from build123d import *

# Parameters (mm, degrees)
SALIENTE_EXTRUIR1_DEPTH = 120
CROQUIS2_R              = 1.5
CORTAR_EXTRUIR1_DEPTH   = 100
CROQUIS3_R              = 1.5
CORTAR_EXTRUIR2_DEPTH   = 100


with BuildPart() as part:
    # Croquis1 → Saliente-Extruir1 (new body)
    with BuildSketch(Plane.XY):
        Polygon((0, 0), (50.8, 0), (50.8, 3.175), (3.175, 3.175), (3.175, 50.8), (0, 50.8), align=None)
    extrude(amount=SALIENTE_EXTRUIR1_DEPTH)

    # Croquis2 → Cortar-Extruir1 (cut)
    with BuildSketch(Plane(origin=(0, 3.175, 0), x_dir=(1, 0, 0), z_dir=(0, 1, 0))):
        with Locations(Location((40.8, -29.9, 0), (0, 0, 180))):
            Circle(CROQUIS2_R)
        with Locations(Location((14.8, -29.9, 0), (0, 0, 180))):
            Circle(CROQUIS2_R)
        with Locations(Location((40.8, -110.1, 0), (0, 0, 180))):
            Circle(CROQUIS2_R)
        with Locations(Location((14.8, -110.1, 0), (0, 0, 180))):
            Circle(CROQUIS2_R)
    extrude(amount=-CORTAR_EXTRUIR1_DEPTH, mode=Mode.SUBTRACT)

    # Croquis3 → Cortar-Extruir2 (cut)
    with BuildSketch(Plane(origin=(0, 3.175, 0), x_dir=(1, 0, 0), z_dir=(0, 1, 0))):
        with Locations(Location((26.985, -6, 0), (0, 0, 180))):
            Circle(CROQUIS3_R)
        with Locations(Location((26.985, -16, 0), (0, 0, 180))):
            Circle(CROQUIS3_R)
    extrude(amount=-CORTAR_EXTRUIR2_DEPTH, mode=Mode.SUBTRACT)


solid = part.part
Source: CAD feature listing. Evaluate the final solid. Frame: model axes, mm. A direction names the side the tool comes from. Round coordinates to 2 decimals unless told otherwise and drop trailing zeros. Loops run counter-clockwise (first coordinate to the right, second up) from the corner with the lowest first, then second, coordinate; pieces in that order, holes last. Notation, with made-up numbers: M -4,-38 L 3,-38 A12 ccw 3,-17 Z; hole C 53,0 d9. An arc over 180 degrees is marked long. Answer as CSV lines item,"result".
Q1. Cut plane A-A (z = 110.1). Return the cut outline in (x, y) (3 decimals).
Verdict:
outline,"M 0,0 L 13.3,0 L 13.3,3.175 L 3.175,3.175 L 3.175,50.8 L 0,50.8 Z; M 16.3,0 L 39.3,0 L 39.3,3.175 L 16.3,3.175 Z; M 42.3,0 L 50.8,0 L 50.8,3.175 L 42.3,3.175 Z"
Q2. Reachability of faces 1 (the face through (3.175, 27, 59)), 2 (the face through (42, 1.6, 109.2)) from +Z, -Z, +X, -X, +Y, -Y: full face, straight path, thin tool, end or side. Return the list, or none.
Verdict:
face 1,"+Z, -Z, +X, +Y"
face 2,"+Y, -Y"
Q3. Line query: line 1 along Z through (x, y) = (14.8, 1.7); line 2 along X through (y, z) = (1, 110); line 3 along Z through (x, y) = (40, 2). Output: solid intervals per line, ascending.
Verdict:
line 1,"z = 0 to 28.4, 31.4 to 108.6, 111.6 to 120"
line 2,"x = 0 to 13.3, 16.3 to 39.3, 42.3 to 50.8"
line 3,"z = 0 to 28.63, 31.17 to 108.83, 111.37 to 120"
Q4. Cut plane D-D (z = 43.5). Return the cut outline in (x, y) (3 decimals).
Verdict:
outline,"M 0,0 L 50.8,0 L 50.8,3.175 L 3.175,3.175 L 3.175,50.8 L 0,50.8 Z"
Q5. Pull-direction query (X, two-part tool) for faces 3 (the face through (0, 26, 59)), 4 (the face through (25.554, 1.61, 6.451)), 5 (the face through (2, 50.8, 59)); classes: +X half, -X half, draft (parallel to the pull), parting line (faces both ways), or undercut.
Verdict:
face 3,"-X half"
face 4,"undercut"
face 5,"draft"
Q6. Cut plane C-C (x = 14.8). Return the cut outline in (y, z) (3 decimals), plus the area to 3 significant figures.
Verdict:
outline,"M 0,0 L 3.175,0 L 3.175,28.4 L 0,28.4 Z; M 0,31.4 L 3.175,31.4 L 3.175,108.6 L 0,108.6 Z; M 0,111.6 L 3.175,111.6 L 3.175,120 L 0,120 Z"
area,"362 mm^2"
Q7. Cut plane B-B (z = 6). Return the cut outline in (x, y) (3 decimals).
Verdict:
outline,"M 0,0 L 25.485,0 L 25.485,3.175 L 3.175,3.175 L 3.175,50.8 L 0,50.8 Z; M 28.485,0 L 50.8,0 L 50.8,3.175 L 28.485,3.175 Z"
Q8. Contact query for flat-ended pins moving along their axis: pin 1 (4 mm diameter, centred on x = 26.985, z = 6, fed in from +Y) (3 decimals); pin 2 (4 mm diameter, centred on y = 40, z = 86, fed in from +X) (3 decimals). Output: stop coordinate, or through.
Verdict:
pin 1,"stops at y = 3.175"
pin 2,"stops at x = 3.175"
